The model under review builds one solid part; all positions refer to its coordinate system, in mm. Face numbers are marked on the shaded views. A direction names the side the tool comes from. Give positions to 0.01 mm unless a question says otherwise; leave off trailing zeros. Order: outer loops, then holes, each group sorted by start corner. A loop starts at its lowest first (then second) coordinate and runs counter-clockwise, first axis right, second up.
```python
from build123d import *

# Parameters (mm, degrees)
F1_DEPTH = 20
F3_DEPTH = 10
F4_START = -10
F2_W     = 60
F2_H     = 13.958594691
F4_DEPTH = 8


with BuildPart() as f1:
    # F0 (on Top) → F1 (new body)
    with BuildSketch(Plane.XY):
        with BuildLine():
            ThreePointArc((-10.1912790055, 32.1777615839), (-15.0978885502, 29.0301175207), (-15.3705234986, 23.207046977))
            Line((-15.3705234986, 23.207046977), (-10.1912790055, 32.1777615839))
        make_face()
        with BuildLine():
            ThreePointArc((-3.2470355891, 25.8546910402), (-4.9020463007, 30.130483236), (-9.0044980948, 32.1777615839))
            Line((-9.0044980948, 32.1777615839), (-3.8252536017, 23.207046977))
            ThreePointArc((-3.8252536017, 23.207046977), (-3.3932737721, 24.4996675021), (-3.2470355891, 25.8546910402))
        make_face()
        with BuildLine():
            Line((-15.9639139539, 22.1792645596), (-15.3705234986, 23.207046977))
            ThreePointArc((-15.3705234986, 23.207046977), (-15.0978885502, 29.0301175207), (-10.1912790055, 32.1777615839))
            Line((-10.1912790055, 32.1777615839), (-9.5978885502, 33.2055440013))
            Line((-9.5978885502, 33.2055440013), (-9.0044980948, 32.1777615839))
            ThreePointArc((-9.0044980948, 32.1777615839), (-4.9020463007, 30.130483236), (-3.2470355891, 25.8546910402))
            ThreePointArc((-3.2470355891, 25.8546910402), (-3.3932737721, 24.4996675021), (-3.8252536017, 23.207046977))
            Line((-3.8252536017, 23.207046977), (-3.2318631464, 22.1792645596))
            Line((-3.2318631464, 22.1792645596), (-4.418644057, 22.1792645596))
            ThreePointArc((-4.418644057, 22.1792645596), (-5.2919075177, 21.1865157348), (-6.351802086, 20.3960963492))
            Line((-6.351802086, 20.3960963492), (-3.0822347841, 20.3960963492))
            ThreePointArc((-3.0822347841, 20.3960963492), (-1.6093637486, 22.9506470505), (-1.0978885502, 25.8546910402))
            ThreePointArc((-1.0978885502, 25.8546910402), (-12.5019325399, 33.8432158418), (-16.1135423163, 20.3960963492))
            Line((-16.1135423163, 20.3960963492), (-12.8439750143, 20.3960963492))
            ThreePointArc((-12.8439750143, 20.3960963492), (-13.9038695826, 21.1865157348), (-14.7771330433, 22.1792645596))
            Line((-14.7771330433, 22.1792645596), (-15.9639139539, 22.1792645596))
        make_face()
        with BuildLine():
            Line((-4.418644057, 22.1792645596), (-14.7771330433, 22.1792645596))
            ThreePointArc((-14.7771330433, 22.1792645596), (-13.9038695826, 21.1865157348), (-12.8439750143, 20.3960963492))
            Line((-12.8439750143, 20.3960963492), (-6.351802086, 20.3960963492))
            ThreePointArc((-6.351802086, 20.3960963492), (-5.2919075177, 21.1865157348), (-4.418644057, 22.1792645596))
        make_face()
    extrude(amount=F1_DEPTH)

    # F0 (on Top) → F3 (join)
    with BuildSketch(Plane.XY):
        with BuildLine():
            ThreePointArc((-10.1912790055, 32.1777615839), (-15.0978885502, 29.0301175207), (-15.3705234986, 23.207046977))
            Line((-15.3705234986, 23.207046977), (-10.1912790055, 32.1777615839))
        make_face()
        Polygon((-9.5978885502, 32.2055440013), (-15.0978885502, 22.6792645596), (-4.0978885502, 22.6792645596), align=None)
        with BuildLine():
            ThreePointArc((-10.1912790055, 32.1777615839), (-9.8949087916, 32.1985945947), (-9.5978885502, 32.2055440013))
            ThreePointArc((-9.5978885502, 32.2055440013), (-9.3008683088, 32.1985945947), (-9.0044980948, 32.1777615839))
            Line((-9.0044980948, 32.1777615839), (-9.5978885502, 33.2055440013))
            Line((-9.5978885502, 33.2055440013), (-10.1912790055, 32.1777615839))
        make_face()
        with BuildLine():
            ThreePointArc((-15.3705234986, 23.207046977), (-15.2403803083, 22.9399663374), (-15.0978885502, 22.6792645596))
            Line((-15.0978885502, 22.6792645596), (-9.5978885502, 32.2055440013))
            ThreePointArc((-9.5978885502, 32.2055440013), (-9.8949087916, 32.1985945947), (-10.1912790055, 32.1777615839))
            Line((-10.1912790055, 32.1777615839), (-15.3705234986, 23.207046977))
        make_face()
        with BuildLine():
            ThreePointArc((-14.7771330433, 22.1792645596), (-14.9433600669, 22.4255121884), (-15.0978885502, 22.6792645596))
            ThreePointArc((-15.0978885502, 22.6792645596), (-15.2403803083, 22.9399663374), (-15.3705234986, 23.207046977))
            Line((-15.3705234986, 23.207046977), (-15.9639139539, 22.1792645596))
            Line((-15.9639139539, 22.1792645596), (-14.7771330433, 22.1792645596))
        make_face()
        with BuildLine():
            Line((-15.9639139539, 22.1792645596), (-15.3705234986, 23.207046977))
            ThreePointArc((-15.3705234986, 23.207046977), (-15.0978885502, 29.0301175207), (-10.1912790055, 32.1777615839))
            Line((-10.1912790055, 32.1777615839), (-9.5978885502, 33.2055440013))
            Line((-9.5978885502, 33.2055440013), (-9.0044980948, 32.1777615839))
            ThreePointArc((-9.0044980948, 32.1777615839), (-4.9020463007, 30.130483236), (-3.2470355891, 25.8546910402))
            ThreePointArc((-3.2470355891, 25.8546910402), (-3.3932737721, 24.4996675021), (-3.8252536017, 23.207046977))
            Line((-3.8252536017, 23.207046977), (-3.2318631464, 22.1792645596))
            Line((-3.2318631464, 22.1792645596), (-4.418644057, 22.1792645596))
            ThreePointArc((-4.418644057, 22.1792645596), (-5.2919075177, 21.1865157348), (-6.351802086, 20.3960963492))
            Line((-6.351802086, 20.3960963492), (-3.0822347841, 20.3960963492))
            ThreePointArc((-3.0822347841, 20.3960963492), (-1.6093637486, 22.9506470505), (-1.0978885502, 25.8546910402))
            ThreePointArc((-1.0978885502, 25.8546910402), (-12.5019325399, 33.8432158418), (-16.1135423163, 20.3960963492))
            Line((-16.1135423163, 20.3960963492), (-12.8439750143, 20.3960963492))
            ThreePointArc((-12.8439750143, 20.3960963492), (-13.9038695826, 21.1865157348), (-14.7771330433, 22.1792645596))
            Line((-14.7771330433, 22.1792645596), (-15.9639139539, 22.1792645596))
        make_face()
        with BuildLine():
            Line((-4.418644057, 22.1792645596), (-14.7771330433, 22.1792645596))
            ThreePointArc((-14.7771330433, 22.1792645596), (-13.9038695826, 21.1865157348), (-12.8439750143, 20.3960963492))
            Line((-12.8439750143, 20.3960963492), (-6.351802086, 20.3960963492))
            ThreePointArc((-6.351802086, 20.3960963492), (-5.2919075177, 21.1865157348), (-4.418644057, 22.1792645596))
        make_face()
        with BuildLine():
            ThreePointArc((-3.2470355891, 25.8546910402), (-4.9020463007, 30.130483236), (-9.0044980948, 32.1777615839))
            Line((-9.0044980948, 32.1777615839), (-3.8252536017, 23.207046977))
            ThreePointArc((-3.8252536017, 23.207046977), (-3.3932737721, 24.4996675021), (-3.2470355891, 25.8546910402))
        make_face()
        with BuildLine():
            ThreePointArc((-9.0044980948, 32.1777615839), (-9.3008683088, 32.1985945947), (-9.5978885502, 32.2055440013))
            Line((-9.5978885502, 32.2055440013), (-4.0978885502, 22.6792645596))
            ThreePointArc((-4.0978885502, 22.6792645596), (-3.9553967921, 22.9399663374), (-3.8252536017, 23.207046977))
            Line((-3.8252536017, 23.207046977), (-9.0044980948, 32.1777615839))
        make_face()
        with BuildLine():
            Line((-4.0978885502, 22.6792645596), (-15.0978885502, 22.6792645596))
            ThreePointArc((-15.0978885502, 22.6792645596), (-14.9433600669, 22.4255121884), (-14.7771330433, 22.1792645596))
            Line((-14.7771330433, 22.1792645596), (-4.418644057, 22.1792645596))
            ThreePointArc((-4.418644057, 22.1792645596), (-4.2524170335, 22.4255121884), (-4.0978885502, 22.6792645596))
        make_face()
        with BuildLine():
            ThreePointArc((-3.8252536017, 23.207046977), (-3.9553967921, 22.9399663374), (-4.0978885502, 22.6792645596))
            ThreePointArc((-4.0978885502, 22.6792645596), (-4.2524170335, 22.4255121884), (-4.418644057, 22.1792645596))
            Line((-4.418644057, 22.1792645596), (-3.2318631464, 22.1792645596))
            Line((-3.2318631464, 22.1792645596), (-3.8252536017, 23.207046977))
        make_face()
    extrude(amount=-F3_DEPTH)

    # F2 (on Top) → F4 (join)
    with BuildSketch(Plane.XY.offset(F4_START)):
        with Locations((-9.5978885502, 27.3753936947)):
            Rectangle(F2_W, F2_H)
    extrude(amount=-F4_DEPTH)


solid = f1.part
```
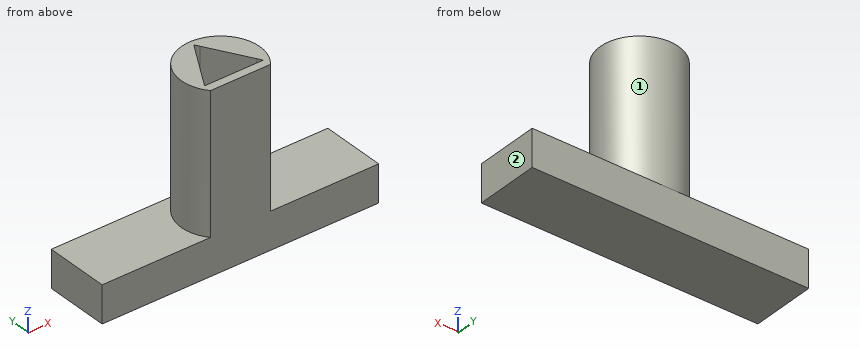
Item 1: Take a section at A-A (y = 27). Give the boundary of the cut face in (x, z), and give its area (3 significant figures).
Values found:
outline: (-39.6, -18) - (20.4, -18) - (20.4, -10) - (-1.18, -10) - (-1.18, 20) - (-6.02, 20) - (-6.02, 0) - (-13.18, 0) - (-13.18, 20) - (-18.02, 20) - (-18.02, -10) - (-39.6, -10) - close
area: 842 mm2
Item 2: Take a section at C-C (x = -4.5). Give the boundary of the cut face in (y, z).
Values found:
outline: (20.4, -18) - (34.35, -18) - (34.35, -10) - (32.66, -10) - (32.66, 20) - (24.38, 20) - (24.38, 0) - (22.18, 0) - (22.18, 20) - (20.4, 20) - close
Item 3: Take a section at B-B (z = 1). Give the boundary of the cut face in (x, y).
Values found:
outline: (-16.11, 20.4) - (-3.08, 20.4) arc R8.5 ccw (long way) to start; hole (-15.96, 22.18) - (-3.23, 22.18) - (-9.6, 33.21) - close
Item 4: For the marked faces 1 and 2, list the 3-axis set-ups (+Z, -Z, +X, -X, +Y, -Y) from which the entire face can be reached by the end or side of a thin tool; tool diameter is ignored.
Values found:
face 1: +Z
face 2: +Z, -Z, +X, +Y, -Y
Item 5: Take a section at D-D (z = -3). Give the boundary of the cut face in (x, y), and give its area (3 significant figures).
Values found:
outline: (-16.11, 20.4) - (-3.08, 20.4) arc R8.5 ccw (long way) to start
area: 199 mm2
Item 6: For line 1 (Z direction, x = 3, y = 21.5); line 2 (X direction, y = 24.25, z = 16.5); line 3 (Z direction, x = -10.5, y = 29.25), list the stretches that pass through material, from the lowest coordinate up.
Values found:
line 1: z = -18 to -10
line 2: x = -17.95 to -14.77, -4.43 to -1.25
line 3: z = -18 to 0
Item 7: Clearance check with flat-ended pins moving along their axes: pin 1 Ø5 at (y, z) = (29, 5.5) entering from +X; pin 2 Ø3 at (x, z) = (-2.5, -4) entering from +Y; pin 3 Ø7 at (x, y) = (9.5, 30) entering from +Z; pin 4 Ø4 at (x, z) = (-20.5, 14) entering from -Y. State where each tip first meets the part, or that it passes through.
Values found:
pin 1: stops at x = -1.12
pin 2: stops at y = 32.25
pin 3: stops at z = -10
pin 4: passes through
